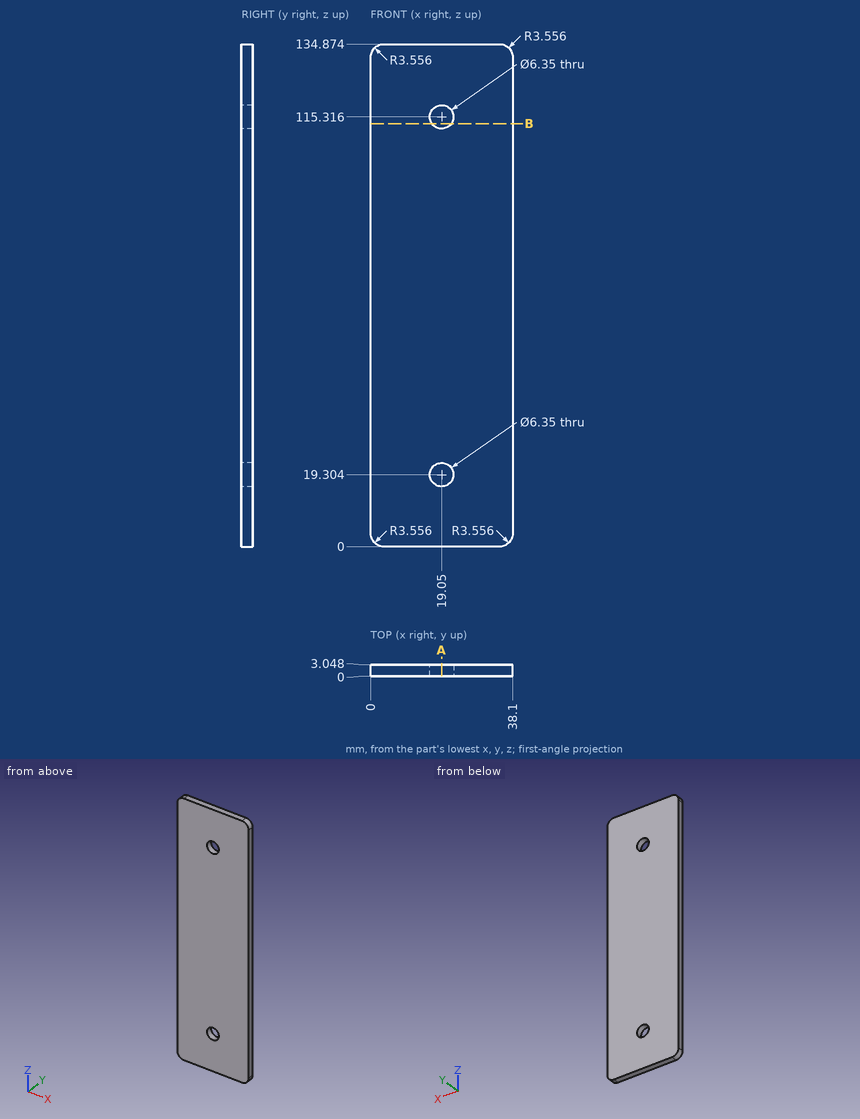
Source: three-view drawing plus pictorial views. Frame: mm from the lowest corner of the part. Give positions to 0.01 mm unless a question says otherwise; leave off trailing zeros. Order: outer loops, then holes, each group sorted by start corner. A loop starts at its lowest first (then second) coordinate and runs counter-clockwise, first axis right, second up. Notation, with made-up numbers: (57, 37) -> (106, 37) arc R31 cw to (106, 63) -> close; hole circle Ø5 at (-16, -25.75). An arc over 180 degrees is marked (long way). Use a Markdown table: item, result.
Q1. Section A-A (x = 19.05). Return the cut outline in (y, z), and give its area (3 significant figures).
A:
| item | result |
|---|---|
| outline | (0, 0) -> (3.05, 0) -> (3.05, 16.13) -> (0, 16.13) -> close; (0, 22.48) -> (3.05, 22.48) -> (3.05, 112.14) -> (0, 112.14) -> close; (0, 118.49) -> (3.05, 118.49) -> (3.05, 134.87) -> (0, 134.87) -> close |
| area | 372 mm^2 |
Q2. Section B-B (z = 113.5). Return the cut outline in (x, y).
A:
| item | result |
|---|---|
| outline | (0, 0) -> (16.45, 0) -> (16.45, 3.05) -> (0, 3.05) -> close; (21.65, 0) -> (38.1, 0) -> (38.1, 3.05) -> (21.65, 3.05) -> close |
Q3. Material intervals for line 1 (Z direction, x = 19.05, y = 1.95); line 2 (Z direction, x = 17, y = 2.9); line 3 (X direction, y = 1.85, z = 17), sorted ascending. Write a range as [from, to].
A:
| item | result |
|---|---|
| line 1 | [0, 16.13], [22.48, 112.14], [118.49, 134.87] |
| line 2 | [0, 16.88], [21.73, 112.89], [117.74, 134.87] |
| line 3 | [0, 16.87], [21.23, 38.1] |
Q4. First-contact query: P1, Ø5, axis at x = 19.05, z = 115.316, coming from the -Y side. Flat tip, straight axial feed; report the tip coordinate or a pass-through.
A:
| item | result |
|---|---|
| P1 | through |
